```python
from build123d import *

# Parameters (mm, degrees)
TUBE008_R         = 15
TUBE008_R_2       = 3.75
TUBE008_DEPTH     = 2
ARRAY002_Z_COUNT  = 3
ARRAY002_Z_PITCH  = 25
TUBE007_R         = 3.75
TUBE007_R_2       = 2.75
TUBE007_DEPTH     = 100
CYLINDER004_R     = 1.5
CYLINDER004_DEPTH = 100
ARRAY001_COUNT    = 5
CYLINDER005_R     = 1.5
CYLINDER005_DEPTH = 10
ARRAY007_COUNT    = 3
TUBE006_R         = 15
TUBE006_R_2       = 2.75
TUBE006_DEPTH     = 5
CYLINDER001_R     = 23.8
CYLINDER001_DEPTH = 3.5
CYLINDER006_R     = 31.9
CYLINDER006_DEPTH = 3.5
CYLINDER_R        = 26.5
CYLINDER_DEPTH    = 3


with BuildPart() as pistonshaftspacers:
    # Tube008 → Tube008 (new body)
    with BuildSketch(Plane.XY.offset(31.5)):
        Circle(TUBE008_R)
        Circle(TUBE008_R_2, mode=Mode.SUBTRACT)
    extrude(amount=TUBE008_DEPTH)

    # Array002 Z: PistonShaftSpacers ×3


with BuildPart() as pistonshaftspacers_1:
    add(pistonshaftspacers.part)
    with Locations(*[(0, 0, i * ARRAY002_Z_PITCH) for i in range(1, ARRAY002_Z_COUNT)]):
        add(pistonshaftspacers.part)


with BuildPart() as pistonshaft:
    # Tube007 → Tube007 (new body)
    with BuildSketch(Plane.XY.offset(10)):
        Circle(TUBE007_R)
        Circle(TUBE007_R_2, mode=Mode.SUBTRACT)
    extrude(amount=TUBE007_DEPTH)


with BuildPart() as obj1:
    # Cylinder004 → Cylinder004 (new body)
    with BuildSketch(Plane(origin=(0, 12, 10), x_dir=(1, 0, 0), z_dir=(0, 0, 1))):
        Circle(CYLINDER004_R)
    extrude(amount=CYLINDER004_DEPTH)

    # Array001: obj1 ×5 about axis
    array001_axis = Axis((0, 0, 0), (0, 0, 1))


with BuildPart() as obj1_1:
    add(obj1.part)
    for i in range(1, ARRAY001_COUNT):
        add(obj1.part.rotate(array001_axis, i * 360 / ARRAY001_COUNT))


with BuildPart() as pistonconnectorscrewcutters:
    # Cylinder005 → Cylinder005 (new body)
    with BuildSketch(Plane(origin=(6.5, 0, 110), x_dir=(1, 0, 0), z_dir=(0, 0, 1))):
        Circle(CYLINDER005_R)
    extrude(amount=CYLINDER005_DEPTH)

    # Array007: PistonConnectorScrewCutters ×3 about axis
    array007_axis = Axis((0, 0, 0), (0, 0, 1))


with BuildPart() as pistonconnectorscrewcutters_1:
    add(pistonconnectorscrewcutters.part)
    for i in range(1, ARRAY007_COUNT):
        add(pistonconnectorscrewcutters.part.rotate(array007_axis, i * 360 / ARRAY007_COUNT))


with BuildPart() as pistonnutconnectorcutted:
    # Tube006 → Tube006 (new body)
    with BuildSketch(Plane.XY.offset(110)):
        Circle(TUBE006_R)
        Circle(TUBE006_R_2, mode=Mode.SUBTRACT)
    extrude(amount=TUBE006_DEPTH)

    # Cut: cut PistonConnectorScrewCutters
    add(pistonconnectorscrewcutters_1.part, mode=Mode.SUBTRACT)


with BuildPart() as pistonbaseinner:
    # Cylinder001 → Cylinder001 (new body)
    with BuildSketch(Plane.XY.offset(3)):
        Circle(CYLINDER001_R)
    extrude(amount=CYLINDER001_DEPTH)


with BuildPart() as pistonguard:
    # Cylinder006 → Cylinder006 (new body)
    with BuildSketch(Plane.XY.offset(6.5)):
        Circle(CYLINDER006_R)
    extrude(amount=CYLINDER006_DEPTH)


with BuildPart() as piston:
    # Cylinder → Cylinder (new body)
    with BuildSketch(Plane.XY):
        Circle(CYLINDER_R)
    extrude(amount=CYLINDER_DEPTH)

    # Fusion005: union PistonBaseInner, PistonGuard
    add(pistonbaseinner.part)
    add(pistonguard.part)

    # Fusion006: union PistonShaftSpacers, PistonShaft, obj1, PistonNutConnectorCutted
    add(pistonshaftspacers_1.part)
    add(pistonshaft.part)
    add(obj1_1.part)
    add(pistonnutconnectorcutted.part)


solid = piston.part
```
Read the model definition and answer for the solid it produces. Units are mm, in the model's axes. A direction names the side the tool comes from. Give positions to 0.01 mm unless a question says otherwise; leave off trailing zeros. Order: outer loops, then holes, each group sorted by start corner. A loop starts at its lowest first (then second) coordinate and runs counter-clockwise, first axis right, second up.
(1) Find section D-D (y = 16.5). Give the vertices of the cut face in (x, z).
(2) Find section B-B (y = -5.5). Give the number of separate pieces and of enclosed holes in the cut face, plus the area to 3 significant figures.
(3) Find section A-A (z = 52). Give the vertices of the cut face in (x, y), plus the area to 3 significant figures.
(4) Given pin 1 (10 mm diameter, centred on x = 0.5, z = 17, fed in from +Y); pin 2 (4 mm diameter, centred on x = -1.5, z = 59.5, fed in from +Y); pin 3 (2.5 mm diameter, centred on x = -3.25, y = 5.63, fed in from +Z); pin 4 (6 mm diameter, centred on x = -20.5, z = 32.5, fed in from +Y), each flat-ended and moving along its own axis, determine where each tip first touches the part or whether it passes through.
(5) Straight lines are drawn through the part: L1, parallel to Z at x = 8.5, y = -4; L2, parallel to Y at x = 0, z = 44; L3, parallel to Y at x = -3.25, z = 111.3. For each, find the intervals that lie inside material, in ascending order.
(6) For faces 1 (the cylindrical face through (14.246, 22.345, 1.479)), 2 (the cylindrical face through (30.427, 9.582, 8.226)), 3 (the flat face through (3, -3, 33.5)), 4 (the cylindrical face through (-14.985, 0.66, 112.465)), determine the directions among +Z, -Z, +X, -X, +Y, -Y from which every point of the face is accessible in a straight line to the end or side of a thin tool.
(7) For a pull along X with two mould halves and no side action, classify faces 5 (the cylindrical face through (10.18, 4.56, 96.56)), 6 (the cylindrical face through (-14.985, 0.66, 32.486)) as released by +X, released by -X, zero draft, split by the parting line, or undercut.
Result sheet:
1. outline: (-27.3, 6.5) - (-17.15, 6.5) - (-17.15, 3) - (-20.74, 3) - (-20.74, 0) - (20.74, 0) - (20.74, 3) - (17.15, 3) - (17.15, 6.5) - (27.3, 6.5) - (27.3, 10) - (-27.3, 10) - close
2. separate pieces: 6
2. enclosed holes: 0
2. area: 830 mm2
3. outline: circle Ø3 at (-11.41, 3.71); circle Ø3 at (-7.05, -9.71); circle Ø7.5 at (0, 0); circle Ø3 at (0, 12); circle Ø3 at (7.05, -9.71); circle Ø3 at (11.41, 3.71); hole circle Ø5.5 at (0, 0)
3. area: 55.8 mm2
4. pin 1: stops at y = 13.5
4. pin 2: stops at y = 15
4. pin 3: stops at z = 83.5
4. pin 4: passes through
5. L1: z = 0 to 10, 31.5 to 33.5, 56.5 to 58.5, 81.5 to 83.5, 110 to 115
5. L2: y = -3.75 to -2.75, 2.75 to 3.75, 10.5 to 13.5
5. L3: y = -14.64 to -7.13, -4.13 to 4.13, 7.13 to 14.64
6. face 1: -Z
6. face 2: +Z, -Z
6. face 3: none
6. face 4: +Z
7. face 5: undercut
7. face 6: split by the parting line
